```python
from build123d import *

# Parameters (mm, degrees)
BASE_FLANGE1_DEPTH                        = 222.25
HOLE_FOR_1_4_SELF_CLINCHING_NUTS_S_SS_C_D = 8.7376
EDGE_FLANGE1_START                        = -228.1555
EDGE_FLANGE1_DEPTH                        = 456.311
SKETCH14_R                                = 3.302
CUT_EXTRUDE2_DEPTH                        = 380.477450424
FILLET1_R                                 = 1.5875
FILLET2_R                                 = 3.175


# Read off the part's stored shape, not the designer's step: Base-Flange1, Edge-Flange1
with BuildPart() as part:
    # Base-Flange1 outline → Base-Flange1 (new body)
    with BuildSketch(Plane(origin=(0, 0, 0), x_dir=(1, 0, 0), z_dir=(0, 1, 0))):
        with BuildLine():
            Line((304.3555, 6.4389), (304.3555, 44.45))
            Line((304.3555, 44.45), (301.0916, 44.45))
            Line((301.0916, 44.45), (301.0916, 6.4389))
            ThreePointArc((301.0916, 6.4389), (300.16166403, 4.19383597), (297.9166, 3.2639))
            Line((297.9166, 3.2639), (-297.9166, 3.2639))
            ThreePointArc((-297.9166, 3.2639), (-300.16166403, 4.19383597), (-301.0916, 6.4389))
            Line((-301.0916, 6.4389), (-301.0916, 44.45))
            Line((-301.0916, 44.45), (-304.3555, 44.45))
            Line((-304.3555, 44.45), (-304.3555, 6.4389))
            ThreePointArc((-304.3555, 6.4389), (-302.469589853, 1.885910147), (-297.9166, 0))
            Line((-297.9166, 0), (297.9166, 0))
            ThreePointArc((297.9166, 0), (302.469589853, 1.885910147), (304.3555, 6.4389))
        make_face()
    extrude(amount=BASE_FLANGE1_DEPTH)

    # Hole for 1/4 Self-clinching Nuts (S,SS,CLS,CLSS)1 (through all)
    with Locations(Plane.ZY.offset(304.3555)):
        with Locations((-22.225, 174.625), (-22.225, 53.975)):
            Hole(HOLE_FOR_1_4_SELF_CLINCHING_NUTS_S_SS_C_D / 2)

    # Edge-Flange1 outline → Edge-Flange1 (add)
    with BuildSketch(Plane.YZ.offset(EDGE_FLANGE1_START)):
        with BuildLine():
            ThreePointArc((-6.2611, 0), (-10.814089853, -1.885910147), (-12.7, -6.4389))
            Line((-12.7, -6.4389), (-12.7, -31.75))
            Line((-12.7, -31.75), (-9.4361, -31.75))
            Line((-9.4361, -31.75), (-9.4361, -6.4389))
            ThreePointArc((-9.4361, -6.4389), (-8.50616403, -4.19383597), (-6.2611, -3.2639))
            Line((-6.2611, -3.2639), (0, -3.2639))
            Line((0, -3.2639), (0, 0))
            Line((0, 0), (-6.2611, 0))
        make_face()
    extrude(amount=EDGE_FLANGE1_DEPTH)

    # Sketch14 → Cut-Extrude2 (cut, through all)
    with BuildSketch(Plane.XY):
        with Locations((0, 222.25)):
            Circle(SKETCH14_R)
    extrude(amount=-CUT_EXTRUDE2_DEPTH, mode=Mode.SUBTRACT)

    # Fillet1
    fillet1_edges = [part.edges().sort_by_distance(p)[0] for p in [
        (-3.302, 222.25, -1.63195),
        (3.302, 222.25, -1.63195),
    ]]
    fillet(fillet1_edges, radius=FILLET1_R)

    # Fillet2
    fillet2_edges = [part.edges().sort_by_distance(p)[0] for p in [
        (-302.72355, 0, -44.45),
        (302.72355, 0, -44.45),
        (-302.72355, 222.25, -44.45),
        (228.1555, 0, -1.63195),
        (-228.1555, 0, -1.63195),
        (228.1555, -11.06805, -31.75),
        (-228.1555, -11.06805, -31.75),
        (302.72355, 222.25, -44.45),
    ]]
    fillet(fillet2_edges, radius=FILLET2_R)


solid = part.part
```
For this review, take the finished solid that the model builds, in its own axes (mm). A direction names the side the tool comes from. Round coordinates to 2 decimals unless told otherwise and drop trailing zeros. Write each loop counter-clockwise with the first axis right and the second up, starting at its lowest first coordinate (ties: lowest second). Pieces come first, ordered by that corner, then holes. Notation, with made-up numbers: (8.25, 11.25) - (18.25, 11.25) arc R17 cw to (18.25, 43.25) - close; hole circle Ø11 at (22, 58.5). An arc over 180 degrees is marked (long way). Use CSV: the item, a comma, the result in double quotes.
1) For faces 1 (the flat face through (4, 106, -3.264)), 2 (the flat face through (278, 0, -2)), 3 (the flat face through (-301.092, 110, -25)), list the 3-axis set-ups (+Z, -Z, +X, -X, +Y, -Y) from which the entire face can be reached by the end or side of a thin tool; tool diameter is ignored.
Conclusion:
face 1,"-Z, +Y"
face 2,"+Z, -Z, +X, -Y"
face 3,"-Z, +Y, -Y"
2) Clearance check with flat-ended pins moving along their axes: pin 1 Ø5 at (y, z) = (-9.5, -19.5) entering from -X; pin 2 Ø3.5 at (x, y) = (103, -11) entering from -Z; pin 3 Ø4 at (x, y) = (-11.5, 182.5) entering from +Z; pin 4 Ø5 at (x, z) = (-121.5, -8.5) entering from +Y. State where each tip first meets the part, or that it passes through.
Conclusion:
pin 1,"stops at x = -228.16"
pin 2,"stops at z = -31.75"
pin 3,"stops at z = 0"
pin 4,"stops at y = -9.41"
3) Add section B-B on x = -152. Write out the cut boundary in (y, z) (3 decimals), and give its area (3 significant figures).
Conclusion:
outline,"(-12.7, -31.75) - (-9.436, -31.75) - (-9.436, -6.439) arc R3.175 cw to (-6.261, -3.264) - (222.25, -3.264) - (222.25, 0) - (-6.261, 0) arc R6.439 ccw to (-12.7, -6.439) - close"
area,"853 mm^2"
4) Add section C-C on x = 258.5. Write out the cut boundary in (y, z).
Conclusion:
outline,"(0, -3.26) - (222.25, -3.26) - (222.25, 0) - (0, 0) - close"
5) The part is to be moulded in two halves that separate along X. For faces 4 (the flat face through (301.092, 110, -26)), 5 (the flat face through (154, 222.25, -1)), 6 (the flat face through (-304.356, 110, -26)), say which applies: pulls with the +X half, pulls with the -X half, needs draft (parallel to the pull), parting line crosses it, or undercut.
Conclusion:
face 4,"undercut"
face 5,"needs draft"
face 6,"pulls with the -X half"
6) Wall thickness on line 1 along X through (y, z) = (119, -11); line 2 along Z through (x, y) = (-133.5, 47.5); line 3 along Y through (x, z) = (-94, -18.5): over which ranges is each line inside the solid? List them lowest first. Write a range as from..to.
Conclusion:
line 1,"x = -304.36..-301.09, 301.09..304.36"
line 2,"z = -3.26..0"
line 3,"y = -12.7..-9.44"
